For this review, use the dimensioned drawing (mm, ordinates from the lowest corner) and the shaded views. Coordinates: 2 decimals unless noted, no trailing zeros. Order: outer loops, then holes, each group sorted by start corner. A loop starts at its lowest first (then second) coordinate and runs counter-clockwise, first axis right, second up. Notation, with made-up numbers: M 64,81 L 107,81 A29 cw 107,108 Z; hole C 1.5,36 d3. An arc over 180 degrees is marked long. Answer in a Markdown table with one row per item.
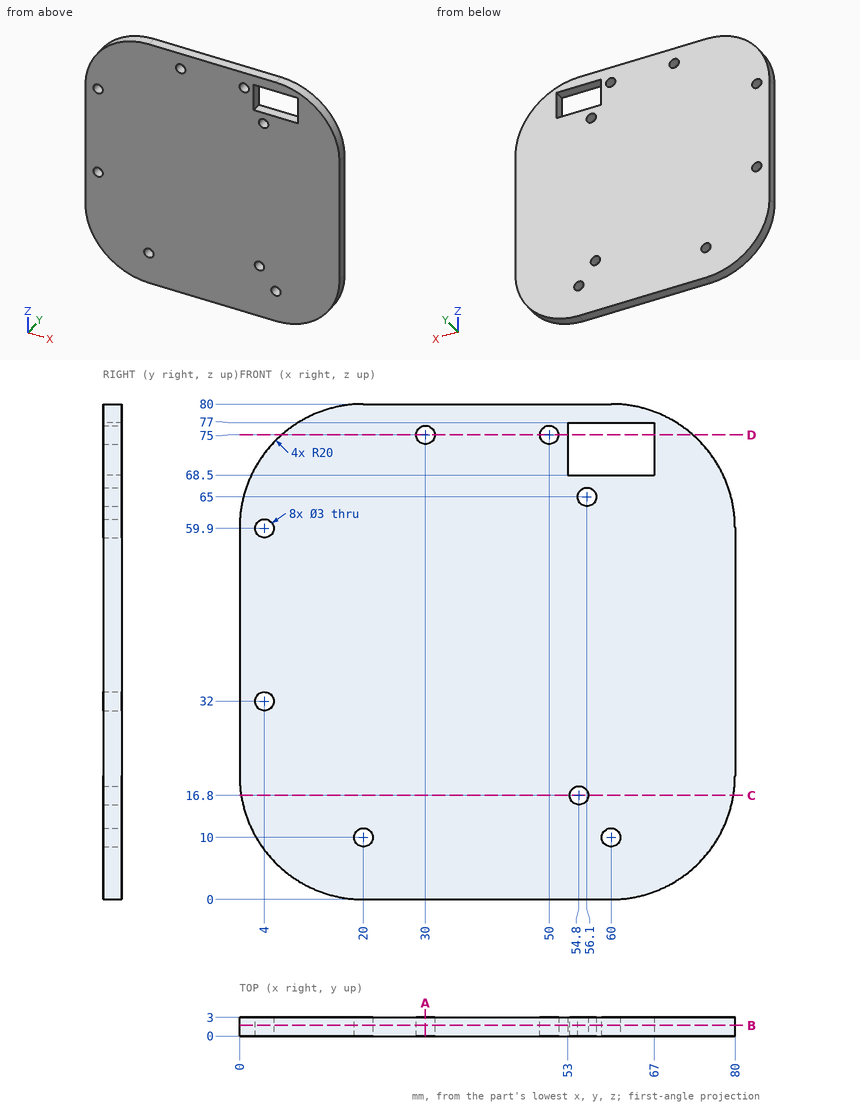
(1) Add section A-A, the plane x = 30. Give the boundary of the cut face in (y, z), and give its area (3 significant figures).
Return value:
| item | result |
|---|---|
| outline | M 0,0 L 3,0 L 3,73.5 L 0,73.5 Z; M 0,76.5 L 3,76.5 L 3,80 L 0,80 Z |
| area | 231 mm2 |
(2) Insertion check: pin 1 Ø0.9 at (y, z) = (2, 73) entering from +X. The pin has a flat end and moves straight along its axis. Give the tip position at first contact, or say it passes through.
Return value:
| item | result |
|---|---|
| pin 1 | stops at x = 75.57 |
(3) Add section D-D, the plane z = 75. Give the boundary of the cut face in (x, y).
Return value:
| item | result |
|---|---|
| outline | M 6.77,0 L 28.5,0 L 28.5,3 L 6.77,3 Z; M 31.5,0 L 48.5,0 L 48.5,3 L 31.5,3 Z; M 51.5,0 L 53,0 L 53,3 L 51.5,3 Z; M 67,0 L 73.23,0 L 73.23,3 L 67,3 Z |
(4) For line 1 along Z through (x, y) = (20, 2.25); line 2 along Z through (x, y) = (56.1, 2.2); line 3 along Z through (x, y) = (4, 1.9), list the stretches that pass through material, from the lowest coordinate up. Write a range as from..to.
Return value:
| item | result |
|---|---|
| line 1 | z = 0..8.5, 11.5..80 |
| line 2 | z = 0..16.05, 17.55..63.5, 66.5..68.5, 77..80 |
| line 3 | z = 8..30.5, 33.5..58.4, 61.4..72 |
(5) Add section C-C, the plane z = 16.8. Give the boundary of the cut face in (x, y).
Return value:
| item | result |
|---|---|
| outline | M 0.26,0 L 53.3,0 L 53.3,3 L 0.26,3 Z; M 56.3,0 L 79.74,0 L 79.74,3 L 56.3,3 Z |
(6) Add section B-B, the plane y = 1.7. Give the number of separate pieces and of enclosed holes in the cut face, and give its area (3 significant figures).
Return value:
| item | result |
|---|---|
| separate pieces | 1 |
| enclosed holes | 9 |
| area | 5,880 mm2 |
